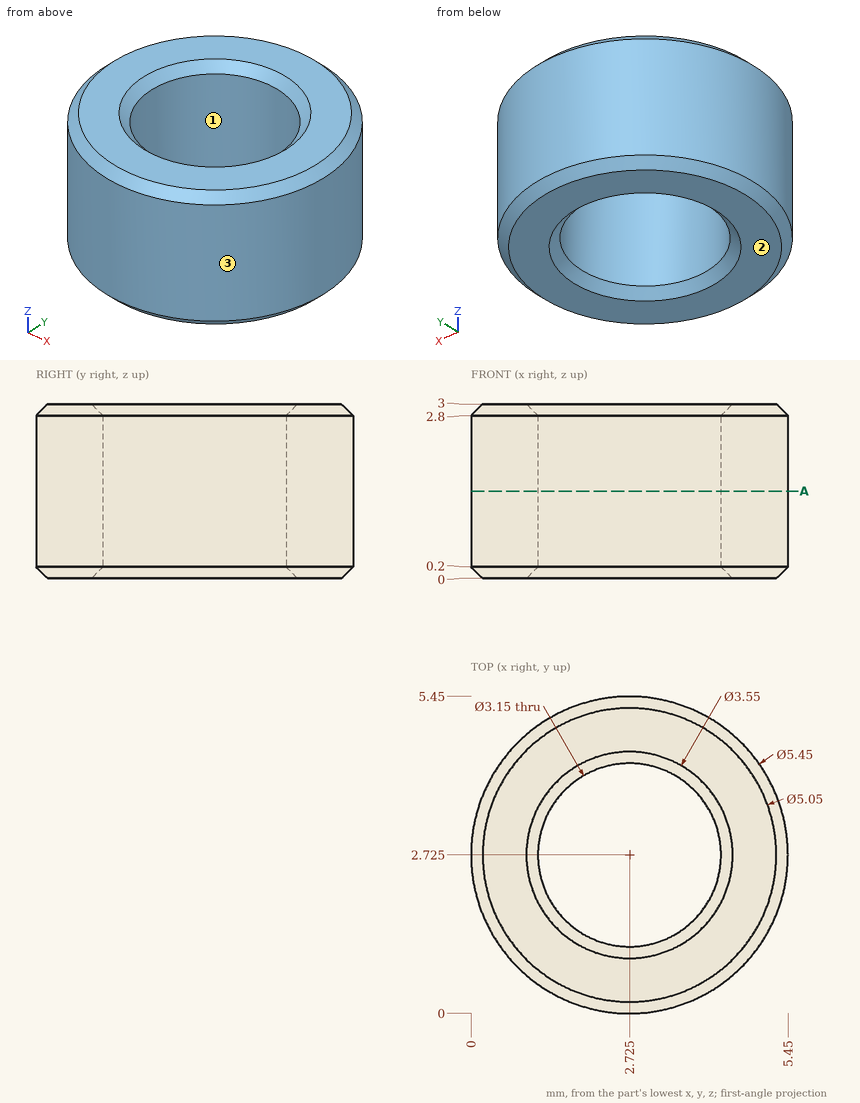
Answer from the drawing. Dimensions are ordinates in mm from the lowest x, y and z of the part. Coordinates: 2 decimals unless noted, no trailing zeros. Loops run counter-clockwise (first coordinate to the right, second up) from the corner with the lowest first, then second, coordinate; pieces in that order, holes last. Notation, with made-up numbers: (6, 47.25) -> (36, 47.25) arc R19 ccw to (36, 57.25) -> close; hole circle Ø8 at (17.5, 86). An arc over 180 degrees is marked (long way). Answer in a Markdown table with one row per item.
Item 1: A cutting plane is placed at A-A on z = 1.5. Determine the outline of the cut face in (x, y) (3 decimals).
Returned:
| item | result |
|---|---|
| outline | circle Ø5.45 at (2.725, 2.725); hole circle Ø3.15 at (2.725, 2.725) |
Item 2: For a pull along Y with two mould halves and no side action, classify the marked faces 1, 2 and 3 as released by +Y, released by -Y, zero draft, split by the parting line, or undercut.
Returned:
| item | result |
|---|---|
| face 1 | undercut |
| face 2 | zero draft |
| face 3 | split by the parting line |
Item 3: Straight lines are drawn through the part: line 1 along X through (y, z) = (2.8, 0.6); line 2 along Y through (x, z) = (1.35, 1.8); line 3 along X through (y, z) = (2.05, 0.45). For each, find the intervals that lie inside material, in ascending order. Write a range as [from, to].
Returned:
| item | result |
|---|---|
| line 1 | x = [0, 1.15], [4.3, 5.45] |
| line 2 | y = [0.37, 1.96], [3.49, 5.08] |
| line 3 | x = [0.08, 1.3], [4.15, 5.37] |
